For this review, take the finished solid that the model builds, in its own axes (mm). Round coordinates to 2 decimals unless told otherwise and drop trailing zeros. Order: outer loops, then holes, each group sorted by start corner. A loop starts at its lowest first (then second) coordinate and runs counter-clockwise, first axis right, second up. Notation, with made-up numbers: M -22,-8 L -18,-8 A5 cw -18,0 Z; hole C -4,24.5 d10. An arc over 180 degrees is marked long. Use a Markdown table: item, result.
from build123d import *

# Parameters (mm, degrees)
F0_R           = 8.255
F1_DEPTH       = 12.7
F3_D           = 5.08
F3_CBORE_D     = 8.255
F3_CBORE_DEPTH = 2.54
F4_R           = 6.35
F5_R           = 25.4


with BuildPart() as f1:
    # F0 (on Right) → F1 (new body)
    with BuildSketch(Plane.YZ):
        Polygon((-27.305, 48.895), (-55.88, -17.78), (166.37, -17.78), (194.945, 48.895), align=None)
        Circle(F0_R, mode=Mode.SUBTRACT)
    extrude(amount=F1_DEPTH)

    # F3 (through all)
    with Locations(Plane(origin=(0, 0, 0), x_dir=(0, -1, 0), z_dir=(-1, 0, 0))):
        with Locations((-175.936093, 40.005), (17.297812, 40.005)):
            CounterBoreHole(F3_D / 2, F3_CBORE_D / 2, F3_CBORE_DEPTH)

    # F4
    f4_edges = [f1.edges().sort_by_distance(p)[0] for p in [
        (6.35, 194.945, 48.895),
        (6.35, -27.305, 48.895),
        (6.35, -55.88, -17.78),
    ]]
    fillet(f4_edges, radius=F4_R)

    # F5
    f5_edges = [f1.edges().sort_by_distance(p)[0] for p in [
        (6.35, 166.37, -17.78),
    ]]
    fillet(f5_edges, radius=F5_R)


solid = f1.part
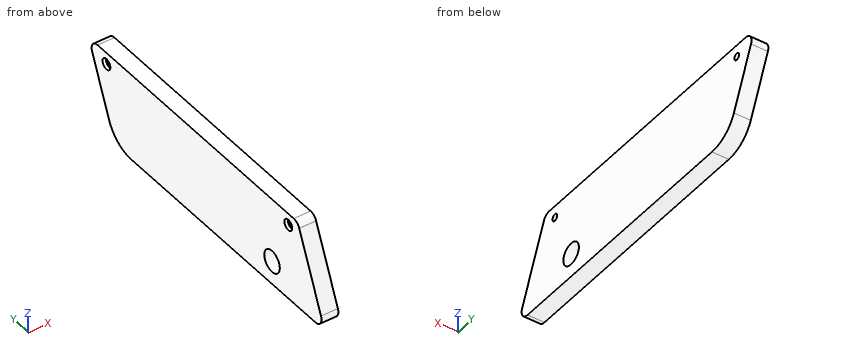
Q1. Add section A-A (z = 0). Write out the cut boundary in (x, y) (3 decimals), then the cut area to 3 significant figures.
Determined:
| item | result |
|---|---|
| outline | M 0,-48.26 L 12.7,-48.26 L 12.7,-8.255 L 0,-8.255 Z; M 0,8.255 L 12.7,8.255 L 12.7,173.99 L 0,173.99 Z |
| area | 2,610 mm^2 |
Q2. Add section B-B (y = 0). Write out the cut boundary in (x, z) (3 decimals), then the cut area to 3 significant figures.
Determined:
| item | result |
|---|---|
| outline | M 0,-17.78 L 12.7,-17.78 L 12.7,-8.255 L 0,-8.255 Z; M 0,8.255 L 12.7,8.255 L 12.7,48.895 L 0,48.895 Z |
| area | 637 mm^2 |
Q3. Wall thickness on line 1 along Y through (x, z) = (6.5, 39.5); line 2 along Z through (x, y) = (7.5, 0) (3 decimals); line 3 along Z through (x, y) = (6.5, -17) (3 decimals): over which ranges is each line inside the solid? List them lowest first. Write a range as [from, to].
Determined:
| item | result |
|---|---|
| line 1 | y = [-31.33, -19.79], [-14.81, 173.45], [178.43, 190.92] |
| line 2 | z = [-17.78, -8.255], [8.255, 48.895] |
| line 3 | z = [-17.78, 37.483], [42.527, 48.895] |
Q4. Clearance check with flat-ended pins moving along their axes: pin 1 (21.5 mm diameter, centred on y = 0, z = 0, fed in from -X); pin 2 (3 mm diameter, centred on x = 3.5, z = 1, fed in from -Y); pin 3 (2 mm diameter, centred on x = 8.5, z = 42, fed in from -Y); pin 4 (8 mm diameter, centred on y = -17.3, z = 40.01, fed in from -X). State where each tip first meets the part, or that it passes through.
Determined:
| item | result |
|---|---|
| pin 1 | stops at x = 0 |
| pin 2 | stops at y = -48.47 |
| pin 3 | stops at y = -30.69 |
| pin 4 | stops at x = 2.54 |
Q5. Add section D-D (y = -35). Write out the cut boundary in (x, z), then the cut area to 3 significant figures.
Determined:
| item | result |
|---|---|
| outline | M 0,-17.78 L 12.7,-17.78 L 12.7,30.94 L 0,30.94 Z |
| area | 619 mm^2 |
Q6. Add section C-C (x = 6.5). Write out the cut boundary in (y, z) (3 decimals).
Determined:
| item | result |
|---|---|
| outline | M -52.087,-8.929 A6.35 ccw -46.25,-17.78 L 149.621,-17.78 A25.4 ccw 172.968,-2.386 L 191.152,40.044 A6.35 ccw 185.315,48.895 L -23.118,48.895 A6.35 ccw -28.954,45.046 Z; hole C -17.298,40.005 d5.08; hole C 0,0 d16.51; hole C 175.936,40.005 d5.08 |
